```python
from build123d import *

# Parameters (mm, degrees)
F1_DEPTH = 2.06
F2_DEPTH = 3.2
F3_DEPTH = 5
F4_DEPTH = 1.4


with BuildPart() as f1:
    # F0 (on Top) → F1 (new body)
    with BuildSketch(Plane.XY):
        with BuildLine():
            ThreePointArc((0, -12.05), (1.803122292, -12.796877708), (2.55, -14.6))
            Line((2.55, -14.6), (4.3422653684, -1.1809874978))
            ThreePointArc((4.3422653684, -1.1809874978), (2.7327235736, -3.5752233315), (0, -4.5))
            Line((0, -4.5), (0, -12.05))
        make_face()
        with BuildLine():
            Line((-0.7071067812, -17.05), (0.7071067812, -17.05))
            ThreePointArc((0.7071067812, -17.05), (2.0378447306, -16.1328694837), (2.55, -14.6))
            ThreePointArc((2.55, -14.6), (1.803122292, -12.796877708), (0, -12.05))
            ThreePointArc((0, -12.05), (-1.803122292, -12.796877708), (-2.55, -14.6))
            ThreePointArc((-2.55, -14.6), (-2.0378447306, -16.1328694837), (-0.7071067812, -17.05))
        make_face()
        with BuildLine():
            ThreePointArc((1.15, -14.6), (-0.8131727984, -15.4131727984), (0, -13.45))
            ThreePointArc((0, -13.45), (0.8131727984, -13.7868272016), (1.15, -14.6))
        make_face(mode=Mode.SUBTRACT)
        with BuildLine():
            Line((-2.55, -3.7077621283), (-2.55, -14.6))
            ThreePointArc((-2.55, -14.6), (-1.803122292, -12.796877708), (0, -12.05))
            Line((0, -12.05), (0, -4.5))
            ThreePointArc((0, -4.5), (-1.335116179, -4.2973788277), (-2.55, -3.7077621283))
        make_face()
        with BuildLine():
            Line((0, 3), (0, 4.5))
            ThreePointArc((0, 4.5), (-2.7327235736, 3.5752233315), (-4.3422653684, 1.1809874978))
            Line((-4.3422653684, 1.1809874978), (-4.5, 0))
            ThreePointArc((-4.5, 0), (-3.9827754142, -2.0946360066), (-2.55, -3.7077621283))
            ThreePointArc((-2.55, -3.7077621283), (-1.335116179, -4.2973788277), (0, -4.5))
            Line((0, -4.5), (0, -3))
            ThreePointArc((0, -3), (-3, 0), (0, 3))
        make_face()
        with BuildLine():
            Line((0, 1.5), (0, 3))
            ThreePointArc((0, 3), (-3, 0), (0, -3))
            Line((0, -3), (0, -1.5))
            ThreePointArc((0, -1.5), (-1.5, 0), (0, 1.5))
        make_face()
        with BuildLine():
            ThreePointArc((-4.3422653684, 1.1809874978), (-2.7327235736, 3.5752233315), (0, 4.5))
            Line((0, 4.5), (0, 12.05))
            ThreePointArc((0, 12.05), (-1.803122292, 12.796877708), (-2.55, 14.6))
            Line((-2.55, 14.6), (-4.3422653684, 1.1809874978))
        make_face()
        with BuildLine():
            ThreePointArc((0, 4.5), (1.335116179, 4.2973788277), (2.55, 3.7077621283))
            Line((2.55, 3.7077621283), (2.55, 14.6))
            ThreePointArc((2.55, 14.6), (1.803122292, 12.796877708), (0, 12.05))
            Line((0, 12.05), (0, 4.5))
        make_face()
        with BuildLine():
            ThreePointArc((2.55, 14.6), (2.0378447306, 16.1328694837), (0.7071067812, 17.05))
            Line((0.7071067812, 17.05), (-0.7071067812, 17.05))
            ThreePointArc((-0.7071067812, 17.05), (-2.0378447306, 16.1328694837), (-2.55, 14.6))
            ThreePointArc((-2.55, 14.6), (-1.803122292, 12.796877708), (0, 12.05))
            ThreePointArc((0, 12.05), (1.803122292, 12.796877708), (2.55, 14.6))
        make_face()
        with BuildLine():
            ThreePointArc((1.15, 14.6), (0.8131727984, 13.7868272016), (0, 13.45))
            ThreePointArc((0, 13.45), (-0.8131727984, 15.4131727984), (1.15, 14.6))
        make_face(mode=Mode.SUBTRACT)
        with BuildLine():
            Line((4.3422653684, -1.1809874978), (4.5, 0))
            ThreePointArc((4.5, 0), (3.9827754142, 2.0946360066), (2.55, 3.7077621283))
            ThreePointArc((2.55, 3.7077621283), (1.335116179, 4.2973788277), (0, 4.5))
            Line((0, 4.5), (0, 3))
            ThreePointArc((0, 3), (2.1213203436, 2.1213203436), (3, 0))
            ThreePointArc((3, 0), (2.1213203436, -2.1213203436), (0, -3))
            Line((0, -3), (0, -4.5))
            ThreePointArc((0, -4.5), (2.7327235736, -3.5752233315), (4.3422653684, -1.1809874978))
        make_face()
        with BuildLine():
            ThreePointArc((3, 0), (2.1213203436, 2.1213203436), (0, 3))
            Line((0, 3), (0, 1.5))
            ThreePointArc((0, 1.5), (1.0606601718, 1.0606601718), (1.5, 0))
            ThreePointArc((1.5, 0), (1.0606601718, -1.0606601718), (0, -1.5))
            Line((0, -1.5), (0, -3))
            ThreePointArc((0, -3), (2.1213203436, -2.1213203436), (3, 0))
        make_face()
    extrude(amount=F1_DEPTH)

    # F0 (on Top) → F2 (join)
    with BuildSketch(Plane.XY):
        with BuildLine():
            Line((0, 1.5), (0, 3))
            ThreePointArc((0, 3), (-3, 0), (0, -3))
            Line((0, -3), (0, -1.5))
            ThreePointArc((0, -1.5), (-1.5, 0), (0, 1.5))
        make_face()
        with BuildLine():
            ThreePointArc((3, 0), (2.1213203436, 2.1213203436), (0, 3))
            Line((0, 3), (0, 1.5))
            ThreePointArc((0, 1.5), (1.0606601718, 1.0606601718), (1.5, 0))
            ThreePointArc((1.5, 0), (1.0606601718, -1.0606601718), (0, -1.5))
            Line((0, -1.5), (0, -3))
            ThreePointArc((0, -3), (2.1213203436, -2.1213203436), (3, 0))
        make_face()
    extrude(amount=F2_DEPTH)

    # F0 (on Top) → F3 (join)
    with BuildSketch(Plane.XY):
        with BuildLine():
            Line((0, 3), (0, 4.5))
            ThreePointArc((0, 4.5), (-2.7327235736, 3.5752233315), (-4.3422653684, 1.1809874978))
            Line((-4.3422653684, 1.1809874978), (-4.5, 0))
            ThreePointArc((-4.5, 0), (-3.9827754142, -2.0946360066), (-2.55, -3.7077621283))
            ThreePointArc((-2.55, -3.7077621283), (-1.335116179, -4.2973788277), (0, -4.5))
            Line((0, -4.5), (0, -3))
            ThreePointArc((0, -3), (-3, 0), (0, 3))
        make_face()
        with BuildLine():
            Line((4.3422653684, -1.1809874978), (4.5, 0))
            ThreePointArc((4.5, 0), (3.9827754142, 2.0946360066), (2.55, 3.7077621283))
            ThreePointArc((2.55, 3.7077621283), (1.335116179, 4.2973788277), (0, 4.5))
            Line((0, 4.5), (0, 3))
            ThreePointArc((0, 3), (2.1213203436, 2.1213203436), (3, 0))
            ThreePointArc((3, 0), (2.1213203436, -2.1213203436), (0, -3))
            Line((0, -3), (0, -4.5))
            ThreePointArc((0, -4.5), (2.7327235736, -3.5752233315), (4.3422653684, -1.1809874978))
        make_face()
    extrude(amount=F3_DEPTH)

    # F0 (on Top) → F4 (cut)
    with BuildSketch(Plane.XY):
        with BuildLine():
            Line((0, 1.5), (0, 3))
            ThreePointArc((0, 3), (-3, 0), (0, -3))
            Line((0, -3), (0, -1.5))
            ThreePointArc((0, -1.5), (-1.5, 0), (0, 1.5))
        make_face()
        with BuildLine():
            ThreePointArc((3, 0), (2.1213203436, 2.1213203436), (0, 3))
            Line((0, 3), (0, 1.5))
            ThreePointArc((0, 1.5), (1.0606601718, 1.0606601718), (1.5, 0))
            ThreePointArc((1.5, 0), (1.0606601718, -1.0606601718), (0, -1.5))
            Line((0, -1.5), (0, -3))
            ThreePointArc((0, -3), (2.1213203436, -2.1213203436), (3, 0))
        make_face()
    extrude(amount=F4_DEPTH, mode=Mode.SUBTRACT)


solid = f1.part
```
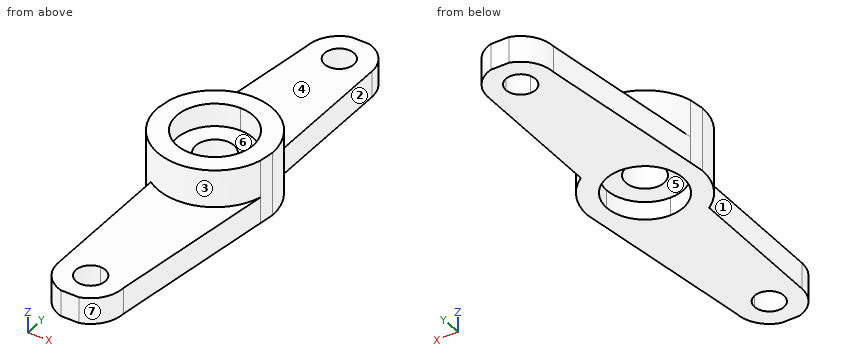
Verification items for the finished model (mm, model axes). Face numbers are marked on the shaded views. A direction names the side the tool comes from. Coordinates: 2 decimals unless noted, no trailing zeros. Loops run counter-clockwise (first coordinate to the right, second up) from the corner with the lowest first, then second, coordinate; pieces in that order, holes last. Notation, with made-up numbers: (-23, -36) - (17, -36) arc R17 cw to (17, -27) - close; hole circle Ø10 at (76, 23.5). An arc over 180 degrees is marked (long way). Answer as a JSON object with one key per item and string values.
(1) Cross-section at B-B, the plane z = 1.1. Record the boundary of the cut face in (x, y), then the cut area to 3 significant figures.
Response:
{"outline": "(-4.5, 0) arc R4.5 ccw to (-2.55, -3.71) - (-2.55, -14.6) arc R2.55 ccw to (-0.71, -17.05) - (0.71, -17.05) arc R2.55 ccw to (2.55, -14.6) - (4.5, 0) arc R4.5 ccw to (2.55, 3.71) - (2.55, 14.6) arc R2.55 ccw to (0.71, 17.05) - (-0.71, 17.05) arc R2.55 ccw to (-2.55, 14.6) - close; hole circle Ø6 at (0, 0); hole circle Ø2.3 at (0, -14.6); hole circle Ø2.3 at (0, 14.6)", "area": "171 mm²"}
(2) Cross-section at D-D, the plane y = -2. Record the boundary of the cut face in (x, z), then the cut area to 3 significant figures.
Response:
{"outline": "(-4.03, 0) - (-2.24, 0) - (-2.24, 1.4) - (2.24, 1.4) - (2.24, 0) - (4.23, 0) - (4.23, 2.06) - (4.03, 2.06) - (4.03, 5) - (2.24, 5) - (2.24, 3.2) - (-2.24, 3.2) - (-2.24, 5) - (-4.03, 5) - close", "area": "26.4 mm²"}
(3) Cross-section at A-A, the plane z = 4.6. Record the boundary of the cut face in (x, y).
Response:
{"outline": "(-4.5, 0) arc R4.5 ccw to (4.34, -1.18) - (4.5, 0) arc R4.5 ccw to (-4.34, 1.18) - close; hole circle Ø6 at (0, 0)"}
(4) Go/stop test with flat-tipped pins: pin 1 Ø4 at (x, y) = (3, -6) entering from +Z; pin 2 Ø1.8 at (x, y) = (0, -14.6) entering from -Z; pin 3 Ø2.5 at (y, z) = (9.5, 1) entering from +X; pin 4 Ø3 at (y, z) = (2, 3) entering from +X. Record where each tip stops, or that it passes through.
Response:
{"pin 1": "stops at z = 2.06", "pin 2": "passes through", "pin 3": "stops at x = 2.55", "pin 4": "stops at x = 4.47"}
(5) Mould release check, pull along X, two halves, no side actions. Record for the marked faces 4, 5, 6 and 7: pulls with the +X half, pulls with the -X half, needs draft (parallel to the pull), parting line crosses it, or undercut.
Response:
{"face 4": "needs draft", "face 5": "undercut", "face 6": "undercut", "face 7": "pulls with the +X half"}
(6) Cross-section at C-C, the plane x = -2.25. Record the boundary of the cut face in (y, z).
Response:
{"outline": "(-15.8, 0) - (-1.98, 0) - (-1.98, 1.4) - (1.98, 1.4) - (1.98, 0) - (15.8, 0) - (15.8, 2.06) - (3.9, 2.06) - (3.9, 5) - (1.98, 5) - (1.98, 3.2) - (-1.98, 3.2) - (-1.98, 5) - (-3.9, 5) - (-3.9, 2.06) - (-15.8, 2.06) - close"}
(7) Scan lines: line 1 along X through (y, z) = (-14.6, 0.8); line 2 along Y through (x, z) = (-2, 0.3); line 3 along Y through (x, z) = (0.5, 3.5). Record each from-to range of solid material in increasing order.
Response:
{"line 1": "x = -2.55 to -1.15, 1.15 to 2.55", "line 2": "y = -16.18 to -2.24, 2.24 to 16.18", "line 3": "y = -4.47 to -2.96, 2.96 to 4.47"}
(8) Access from +Z, -Z, +X, -X, +Y, -Y to the whole of each face (thin tool, end or side, straight path). Record for the marked faces 1, 2 and 3.
Response:
{"face 1": "+Z, -Z, -X, -Y", "face 2": "+Z, -Z, +X, +Y", "face 3": "+Z, -Y"}
